Can you work these out from the model? Positions are in its coordinate system, mm. Face numbers are marked on the shaded views. A direction names the side the tool comes from. Give positions to 0.01 mm unless a question says otherwise; leave off trailing zeros. Write each loop counter-clockwise with the first axis right and the second up, starting at its lowest first coordinate (ties: lowest second). Pieces come first, ordered by that corner, then holes. Notation, with made-up numbers: M 0,68 L 20,68 A7 cw 20,80 Z; hole C 41,-4 d7. An arc over 180 degrees is marked long. Write each question's results on one line, items separated by ' | '.
from build123d import *

# Parameters (mm, degrees)
RESSALTO_EXTRUS_O1_DEPTH = 15
ESBO_O2_W                = 40
ESBO_O2_H                = 3
ESBO_O2_W_2              = 3
ESBO_O2_H_2              = 40
CORTE_EXTRUS_O1_DEPTH    = 13.1
CHANFRO2_SIZE            = 2.5


with BuildPart() as part:
    # Esboço1 → Ressalto-extrusão1 (new body)
    with BuildSketch(Plane.XY):
        Polygon((2.5, 4.5), (2.5, 20), (-2.5, 20), (-2.5, 4.5), (-4.5, 2.5), (-20, 2.5), (-20, -2.5), (-4.5, -2.5), (-2.5, -4.5), (-2.5, -20), (2.5, -20), (2.5, -4.5), (4.5, -2.5), (20, -2.5), (20, 2.5), (4.5, 2.5), align=None)
    extrude(amount=RESSALTO_EXTRUS_O1_DEPTH)

    # Esboço2 → Corte-extrusão1 (cut)
    with BuildSketch(Plane.XY.offset(15)):
        Rectangle(ESBO_O2_W, ESBO_O2_H)
        Rectangle(ESBO_O2_W_2, ESBO_O2_H_2)
    extrude(amount=-CORTE_EXTRUS_O1_DEPTH, mode=Mode.SUBTRACT)

    # Chanfro2
    chanfro2_edges = [part.edges().sort_by_distance(p)[0] for p in [
        (-1.5, -1.5, 8.45),
        (1.5, 1.5, 8.45),
        (-1.5, 1.5, 8.45),
        (1.5, -1.5, 8.45),
    ]]
    chamfer(chanfro2_edges, length=CHANFRO2_SIZE)


solid = part.part
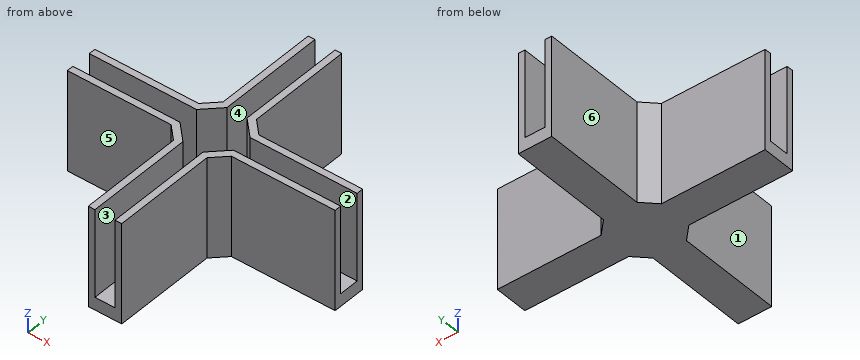
Item 1: I want a section at A-A, the plane z = 5.75. Give the number of separate pieces and of enclosed holes in the cut face, and give its area (4 significant figures).
Geometry says:
separate pieces: 4 | enclosed holes: 0 | area: 139.5 mm2
Item 2: If I drill on line 1 (Y direction, x = -15.5, z = 12.75); line 2 (X direction, y = -15, z = 1), over which ranges is the centre line in solid material (lowest first)? Write a range as from..to.
Geometry says:
line 1: y = -2.5..-1.5, 1.5..2.5 | line 2: x = -2.5..2.5
Item 3: Thinking about a two-plate mould opening in X: for the marked faces 1, 2 and 3, which applies, +X half, -X half, draft (parallel to the pull), parting line (faces both ways), or undercut?
Geometry says:
face 1: -X half | face 2: draft | face 3: undercut
Item 4: For the marked faces 4, 5 and 6, which set-ups out of +Z, -Z, +X, -X, +Y, -Y let a thin tool reach every point of the face, with its end or its side?
Geometry says:
face 4: +Z, +Y, -Y | face 5: +Z, -Z, -X, -Y | face 6: +Z, -Z, -X, +Y
Item 5: I'm going to push flat-ended pins straight in: pin 1 (5 mm diameter, centred on x = 6.5, y = 13.5, fed in from +Z); pin 2 (4 mm diameter, centred on y = -13.5, z = 8, fed in from -X); pin 3 (4 mm diameter, centred on x = 15.5, z = 11, fed in from -Y); pin 4 (7.5 mm diameter, centred on y = 10, z = 6.5, fed in from +X). Where does each tip first touch, or does it pass through?
Geometry says:
pin 1: passes through | pin 2: stops at x = -2.5 | pin 3: stops at y = -2.5 | pin 4: stops at x = 2.5
Item 6: I want a section at B-B, the plane x = 14. Please give me the cut outline in (y, z), and give its area (3 significant figures).
Geometry says:
outline: M -2.5,0 L 2.5,0 L 2.5,15 L 1.5,15 L 1.5,1.9 L -1.5,1.9 L -1.5,15 L -2.5,15 Z | area: 35.7 mm2
